```python
from build123d import *

# Parameters (mm, degrees)
DODANIE_WYCI_GNI_CIE1_DEPTH     = 0.35
DODANIE_WYCI_GNI_CIE2_DEPTH     = 3.4
WYTNIJ_WYCI_GNI_CIE1_DEPTH      = 12.253852902
WYTNIJ_WYCI_GNI_CIE1_DEPTH_BACK = 12.253852902
SZKIC3_W                        = 1.55
SZKIC3_H                        = 1.5
KONWERTUJ_BRY_1_DEPTH           = 3.4
KONWERTUJ_BRY_1_2_DEPTH         = 3.4
DODANIE_WYCI_GNI_CIE3_DEPTH     = 1
DODANIE_WYCI_GNI_CIE4_START     = -1.7
DODANIE_WYCI_GNI_CIE4_DEPTH     = 3.6
WYTNIJ_WYCI_GNI_CIE2_DEPTH      = 13.252457687


# Read off the part's stored shape, not the designer's step: Konwertuj bryłę1
with BuildPart() as part:
    # Szkic1 → Dodanie-wyciągnięcie1 (new body)
    with BuildSketch(Plane.XY):
        with BuildLine():
            Line((3.5, 0), (3.5, 3.4))
            Line((3.5, 3.4), (3.1, 3.4))
            Line((3.1, 3.4), (2.269798394, 3.4))
            ThreePointArc((2.269798394, 3.4), (2.019798394, 3.15), (1.769798394, 3.4))
            Line((1.769798394, 3.4), (1.417144432, 5.4))
            Line((1.417144432, 5.4), (-1.417144432, 5.4))
            Line((-1.417144432, 5.4), (-1.769798394, 3.4))
            ThreePointArc((-1.769798394, 3.4), (-2.019798394, 3.15), (-2.269798394, 3.4))
            Line((-2.269798394, 3.4), (-3.1, 3.4))
            Line((-3.1, 3.4), (-3.5, 3.4))
            Line((-3.5, 3.4), (-3.5, 0))
            Line((-3.5, 0), (-3.1, 0))
            Line((-3.1, 0), (3.1, 0))
            Line((3.1, 0), (3.5, 0))
        make_face()
    extrude(amount=DODANIE_WYCI_GNI_CIE1_DEPTH)

    # Szkic2 → Dodanie-wyciągnięcie2 (add)
    with BuildSketch(Plane.XZ):
        with BuildLine():
            Line((3.15, -5.046862694), (3.15, -6.546862697))
            ThreePointArc((3.15, -6.546862697), (3.164222396, -6.676726465), (3.206215328, -6.800433654))
            Line((3.206215328, -6.800433654), (3.227865546, -6.846862697))
            Line((3.227865546, -6.846862697), (3.614047818, -6.846862697))
            Line((3.614047818, -6.846862697), (3.523423053, -6.652517262))
            ThreePointArc((3.523423053, -6.652517262), (3.505925998, -6.6009726), (3.5, -6.546862697))
            Line((3.5, -6.546862697), (3.5, -5.046862694))
            Line((3.5, -5.046862694), (3.5, -4.746862694))
            Line((3.5, -4.746862694), (3.5, -0.046862697))
            Line((3.5, -0.046862697), (3.5, 0))
            Line((3.5, 0), (3.15, 0))
            Line((3.15, 0), (3.15, -0.046862697))
            Line((3.15, -0.046862697), (3.15, -4.746862694))
            Line((3.15, -4.746862694), (3.15, -5.046862694))
        make_face()
    dodanie_wyci_gni_cie2 = extrude(amount=-DODANIE_WYCI_GNI_CIE2_DEPTH)

    # Lustro1: Dodanie-wyciągnięcie2 across plane
    add(dodanie_wyci_gni_cie2.mirror(Plane(origin=(0, 0, 0), x_dir=(0, 0, 1), z_dir=(1, 0, 0))))

    # Szkic3 → Wytnij-wyciągnięcie1 (cut, two sides: drawn at the far end of the back side and taken through both)
    with BuildSketch(Plane(origin=(3.5, 0, 0), x_dir=(0, 0, -1), z_dir=(1, 0, 0)).offset(-WYTNIJ_WYCI_GNI_CIE1_DEPTH_BACK)):
        with Locations((1.834568124, 1.7)):
            Rectangle(SZKIC3_W, SZKIC3_H)
        Polygon((6.85, 2.4), (6.655654565, 2.4), (6.55, 2.4), (6.546862697, 2.4), (6.546862697, 0), (4.749999997, 0), (4.618517663, -2.046100673), (8.285753876, -1.25448224), align=None)
        Polygon((6.546862697, 0), (6.546862697, 2.4), (5.049999997, 2.4), (5.049999997, 0.3), (4.749999997, 0), align=None)
    extrude(amount=WYTNIJ_WYCI_GNI_CIE1_DEPTH + WYTNIJ_WYCI_GNI_CIE1_DEPTH_BACK, mode=Mode.SUBTRACT)

    # Konwertuj bryłę1 outline → Konwertuj bryłę1 (cut)
    with BuildSketch(Plane(origin=(0, 0, 0), x_dir=(1, 0, 0), z_dir=(0, 1, 0))):
        with BuildLine():
            Line((3.15, 6.546862697), (3.5, 6.546862697))
            ThreePointArc((3.5, 6.546862697), (3.505925998, 6.6009726), (3.523423053, 6.652517262))
            Line((3.523423053, 6.652517262), (3.614047818, 6.846862697))
            Line((3.614047818, 6.846862697), (3.227865546, 6.846862697))
            Line((3.227865546, 6.846862697), (3.206215328, 6.800433654))
            ThreePointArc((3.206215328, 6.800433654), (3.164222396, 6.676726465), (3.15, 6.546862697))
        make_face()
        with BuildLine():
            Line((3.5, -0.35), (3.5, 0.2))
            ThreePointArc((3.5, 0.2), (3.33890873, -0.18890873), (2.95, -0.35))
            Line((2.95, -0.35), (3.5, -0.35))
        make_face()
        with BuildLine():
            Line((-3.5, -0.35), (-2.95, -0.35))
            ThreePointArc((-2.95, -0.35), (-3.33890873, -0.18890873), (-3.5, 0.2))
            Line((-3.5, 0.2), (-3.5, -0.35))
        make_face()
        with BuildLine():
            ThreePointArc((-3.523423053, 6.652517262), (-3.505925998, 6.6009726), (-3.5, 6.546862697))
            Line((-3.5, 6.546862697), (-3.15, 6.546862697))
            ThreePointArc((-3.15, 6.546862697), (-3.164222396, 6.676726465), (-3.206215328, 6.800433654))
            Line((-3.206215328, 6.800433654), (-3.227865546, 6.846862697))
            Line((-3.227865546, 6.846862697), (-3.614047818, 6.846862697))
            Line((-3.614047818, 6.846862697), (-3.523423053, 6.652517262))
        make_face()
    extrude(amount=KONWERTUJ_BRY_1_DEPTH, mode=Mode.SUBTRACT)

    # Konwertuj bry_1 2 outline → Konwertuj bry_1 2 (add)
    with BuildSketch(Plane(origin=(0, 0, 0), x_dir=(1, 0, 0), z_dir=(0, 1, 0))):
        with BuildLine():
            Line((3.15, 0), (3.15, 0.2))
            ThreePointArc((3.15, 0.2), (3.091421356, 0.058578644), (2.95, 0))
            Line((2.95, 0), (3.15, 0))
        make_face()
        with BuildLine():
            Line((-3.15, 0), (-2.95, 0))
            ThreePointArc((-2.95, 0), (-3.091421356, 0.058578644), (-3.15, 0.2))
            Line((-3.15, 0.2), (-3.15, 0))
        make_face()
    extrude(amount=KONWERTUJ_BRY_1_2_DEPTH)

    # Szkic8 → Dodanie-wyciągnięcie3 (add)
    with BuildSketch(Plane.XZ.offset(-2.4)):
        with BuildLine():
            Line((3.206215328, -6.800433654), (3.227865546, -6.846862697))
            Line((3.227865546, -6.846862697), (3.614047818, -6.846862697))
            Line((3.614047818, -6.846862697), (3.523423053, -6.652517262))
            ThreePointArc((3.523423053, -6.652517262), (3.505925998, -6.6009726), (3.5, -6.546862697))
            Line((3.5, -6.546862697), (3.15, -6.546862697))
            ThreePointArc((3.15, -6.546862697), (3.164222396, -6.676726465), (3.206215328, -6.800433654))
        make_face()
    dodanie_wyci_gni_cie3 = extrude(amount=-DODANIE_WYCI_GNI_CIE3_DEPTH)

    # Lustro2: Dodanie-wyciągnięcie3 across plane
    add(dodanie_wyci_gni_cie3.mirror(Plane(origin=(0, 0, 0), x_dir=(0, 0, 1), z_dir=(1, 0, 0))))

    # Szkic9 → Dodanie-wyciągnięcie4 (add)
    with BuildSketch(Plane(origin=(3.5, 0, 0), x_dir=(0, 0, -1), z_dir=(1, 0, 0)).offset(DODANIE_WYCI_GNI_CIE4_START)):
        with BuildLine():
            Line((2.159795211, 8.048412492), (2.159795211, 9.233988579))
            Line((2.159795211, 9.233988579), (1.809795211, 9.233988579))
            Line((1.809795211, 9.233988579), (1.809795211, 8.048412492))
            Line((1.809795211, 8.048412492), (1.809795211, 7.974008773))
            ThreePointArc((1.809795211, 7.974008773), (1.783153047, 7.840069572), (1.707282584, 7.7265214))
            Line((1.707282584, 7.7265214), (-0.159619408, 5.859619408))
            ThreePointArc((-0.159619408, 5.859619408), (-0.300521696, 5.648744231), (-0.35, 5.4))
            Line((-0.35, 5.4), (-0.35, 3.4))
            Line((-0.35, 3.4), (0, 3.4))
            Line((0, 3.4), (0, 5.4))
            ThreePointArc((0, 5.4), (0.02283614, 5.51480503), (0.087867966, 5.612132034))
            Line((0.087867966, 5.612132034), (1.954769957, 7.479034026))
            ThreePointArc((1.954769957, 7.479034026), (2.106510883, 7.70613037), (2.159795211, 7.974008773))
            Line((2.159795211, 7.974008773), (2.159795211, 8.048412492))
        make_face()
    extrude(amount=-DODANIE_WYCI_GNI_CIE4_DEPTH)

    # Szkic10 → Wytnij-wyciągnięcie2 (cut, through all)
    with BuildSketch(Plane.XY.offset(0.35)):
        with BuildLine():
            Line((-1.8, 5.4), (-1.414602313, 5.4))
            add(Edge.make_bspline(
                [(-1.349117856, 5.857315964), (-1.37109798, 5.736696856), (-1.392626241, 5.570542489), (-1.414602313, 5.4)],
                knots=[0, 0, 0, 0, 0.995518499, 0.995518499, 0.995518499, 0.995518499], degree=3))
            Line((-1.349117856, 5.857315964), (-0.883579694, 7.724217956))
            add(Edge.make_bspline(
                [(-0.810874078, 7.971705329), (-0.835264826, 7.87948746), (-0.859188951, 7.789425824), (-0.883579694, 7.724217956)],
                knots=[0, 0, 0, 0, 1, 1, 1, 1], degree=3))
            Line((-0.810874078, 7.971705329), (-0.797754695, 8.04610905))
            Line((-0.797754695, 8.04610905), (-0.797754695, 9.231685135))
            Line((-0.797754695, 9.231685135), (-0.993203543, 9.461775101))
            Line((-0.993203543, 9.461775101), (-2.257838498, 9.461775101))
            Line((-2.257838498, 9.461775101), (-2.100122127, 3.339055662))
            Line((-2.100122127, 3.339055662), (-1.769812995, 3.397298074))
            ThreePointArc((-1.769812995, 3.397298074), (-1.769802044, 3.398649017), (-1.769798394, 3.4))
            Line((-1.769798394, 3.4), (-1.8, 3.4))
            Line((-1.8, 3.4), (-1.8, 5.4))
        make_face()
        with BuildLine():
            Line((1.8, 5.4), (1.8, 3.47771191))
            Line((1.8, 3.47771191), (2.752350462, 6.206517892))
            Line((2.752350462, 6.206517892), (2.752350462, 10.079155902))
            Line((2.752350462, 10.079155902), (0.802245305, 9.231685135))
            Line((0.802245305, 9.231685135), (0.802245305, 8.04568496))
            Line((0.802245305, 8.04568496), (0.815154302, 7.972474402))
            add(Edge.make_bspline(
                [(0.888230882, 7.723724279), (0.863715686, 7.789264869), (0.839669493, 7.879786029), (0.815154302, 7.972474402)],
                knots=[0, 0, 0, 0, 1, 1, 1, 1], degree=3))
            Line((0.888230882, 7.723724279), (1.353548426, 5.857707011))
            add(Edge.make_bspline(
                [(1.419093822, 5.4), (1.3970978, 5.570696055), (1.375549103, 5.736975116), (1.353548426, 5.857707011)],
                knots=[0.005151663, 0.005151663, 0.005151663, 0.005151663, 1, 1, 1, 1], degree=3))
            Line((1.419093822, 5.4), (1.8, 5.4))
        make_face()
    extrude(amount=-WYTNIJ_WYCI_GNI_CIE2_DEPTH, mode=Mode.SUBTRACT)


solid = part.part
```
Geometry check sheet. Reference: the model listing, model coordinates, mm. A direction names the side the tool comes from. Give positions to 0.01 mm unless a question says otherwise; leave off trailing zeros. Order: outer loops, then holes, each group sorted by start corner. A loop starts at its lowest first (then second) coordinate and runs counter-clockwise, first axis right, second up. Notation, with made-up numbers: (34, 30) - (75, 30) arc R36 cw to (75, 65) - close; hole circle Ø10 at (-37, -11.5). An arc over 180 degrees is marked (long way). Write item = value, one per line. Start each with the question number.
1) Scan lines: L1, parallel to X at y = 1, z = -3; L2, parallel to Z at x = 0.25, y = 0.75; L3, parallel to Y at x = 3.25, z = -0.5. Record each from-to range of solid material in increasing order.
2) Gauge pin test, flat ends, axial feed: pin 1 Ø0.5 at (x, z) = (3.5, -6) entering from -Y; pin 2 Ø0.6 at (x, y) = (0, 8.5) entering from -Z; pin 3 Ø2 at (y, z) = (1.5, -2) entering from +X; pin 4 Ø0.7 at (x, z) = (2.5, -2.5) entering from +Y. Record the tip position at first contact, or that the pin passes through.
3) Section check C-C (x = 0.25). Enter the section's corners in (y, z).
4) Draft check along X on faces 1 (the flat face through (3.34, 3.4, -3.23)), 2 (the flat face through (-3.15, 2, -3)), 3 (the flat face through (1.137, 6.726, -0.971)). Enter one of: released by +X, released by -X, zero draft, split by the parting line, or undercut.
5) Section check B-B (z = -1.5). Enter the section's corners in (x, y).
6) Section check D-D (z = -0.5). Enter the section's corners in (x, y), then the cut area to 3 significant figures.
7) Access from +Z, -Z, +X, -X, +Y, -Y to the whole of each face (thin tool, end or side, straight path). Record for faces 4 (the flat face through (-3.5, 2, -3)), 5 (the flat face through (0, 9, -1.81)), 6 (the flat face through (0, 2, 0)), 7 (the flat face through (3.5, 2, -3)), 8 (the flat face through (3.15, 2, -3)).
8) Section check A-A (z = -2.75). Enter the section's corners in (x, y), then the cut area to 3 significant figures.
Geometry check:
q1.L1 = -3.5 to -3.15, 3.15 to 3.5
q1.L2 = 0 to 0.35
q1.L3 = 0 to 3.4
q2.pin_1 = 2.4
q2.pin_2 = -2.16
q2.pin_3 = 3.5
q2.pin_4 = through
q3.outline = (0, 0) - (5.4, 0) arc R0.3 cw to (5.61, -0.09) - (7.48, -1.95) arc R0.7 ccw to (7.97, -2.16) - (9.23, -2.16) - (9.23, -1.81) - (7.97, -1.81) arc R0.35 cw to (7.73, -1.71) - (5.86, 0.16) arc R0.65 ccw to (5.4, 0.35) - (0, 0.35) - close
q4.face_1 = zero draft
q4.face_2 = undercut
q4.face_3 = released by +X
q5.outline = (-3.5, 0) - (-3.15, 0) - (-3.15, 0.95) - (-3.5, 0.95) - close; (-3.5, 2.45) - (-3.15, 2.45) - (-3.15, 3.4) - (-3.5, 3.4) - close; (-1.06, 7.02) - (1.06, 7.02) - (0.94, 7.52) - (-0.93, 7.52) - close; (3.15, 0) - (3.5, 0) - (3.5, 0.95) - (3.15, 0.95) - close; (3.15, 2.45) - (3.5, 2.45) - (3.5, 3.4) - (3.15, 3.4) - close
q6.outline = (-3.5, 0) - (-3.15, 0) - (-3.15, 3.4) - (-3.5, 3.4) - close; (-1.31, 6.02) - (1.31, 6.02) - (1.19, 6.52) - (-1.18, 6.52) - close; (3.15, 0) - (3.5, 0) - (3.5, 3.4) - (3.15, 3.4) - close
q6.area = 3.62 mm2
q7.face_4 = +Z, -X, +Y, -Y
q7.face_5 = +Z, +X, -X, +Y
q7.face_6 = -Z, -Y
q7.face_7 = +Z, +X, +Y, -Y
q7.face_8 = -Z, +Y, -Y
q8.outline = (-3.5, 0) - (-3.15, 0) - (-3.15, 3.4) - (-3.5, 3.4) - close; (3.15, 0) - (3.5, 0) - (3.5, 3.4) - (3.15, 3.4) - close
q8.area = 2.38 mm2
